The listing builds one solid part. Answer for the finished solid, in the listing's coordinates (mm). Round coordinates to 2 decimals unless told otherwise and drop trailing zeros. Put each result on its own line as item: value. Start each with the question number.
(1) Section A-A, the plane z = 999 is taken. Count the separate pieces of the cut face and the enclosed holes in it, then the cut area to 3 significant figures.
(2) Straight lines are drawn through the part: line 1 (Y direction, x = 27.4, z = 1000); line 2 (X direction, y = -50, z = 1000.5); line 3 (Y direction, x = -28, z = 999.65). For each, find the intervals that lie inside material, in ascending order.
(3) A flat-ended cylindrical pin translates along its axis: P1, Ø2, axis at x = 27.4, y = 15.47, coming from the -Z side. Find the tip coordinate at first contact, or state that the pin passes through.
```python
from build123d import *

# Parameters (mm, degrees)
CROQUIS1_W              = 110.308657865
CROQUIS1_H              = 110.308657866
CROQUIS1_R              = 3
SALIENTE_EXTRUIR1_DEPTH = 3
CROQUIS3_R              = 1.35
CORTAR_EXTRUIR1_DEPTH   = 4
SKETCH2_R               = 1.55575
CUT_EXTRUDE1_DEPTH      = 4
SKETCH1_R               = 1.1
CUT_EXTRUDE2_DEPTH      = 4


with BuildPart() as part:
    # Croquis1 → Saliente-Extruir1 (new body)
    with BuildSketch(Plane(origin=(25.025391454, -7.129133069, 1001.5), x_dir=(1, 0, 0), z_dir=(0, 0, 1))):
        with Locations((-25.025391455, 7.129133069)):
            Rectangle(CROQUIS1_W, CROQUIS1_H)
        with Locations((-74.389051931, 56.197819511)):
            Circle(CROQUIS1_R, mode=Mode.SUBTRACT)
        with Locations((24.605897435, -42.797129855)):
            Circle(CROQUIS1_R, mode=Mode.SUBTRACT)
        with Locations((-74.389051931, -42.797129855)):
            Circle(CROQUIS1_R, mode=Mode.SUBTRACT)
        with Locations((24.605897435, 56.197819511)):
            Circle(CROQUIS1_R, mode=Mode.SUBTRACT)
    extrude(amount=-SALIENTE_EXTRUIR1_DEPTH)

    # Croquis3 → Cortar-Extruir1 (cut, through all)
    with BuildSketch(Plane(origin=(25.025391454, -7.129133069, 998.5), x_dir=(-1, 0, 0), z_dir=(0, 0, -1))):
        with Locations((37.910718234, 21.399287334)):
            Circle(CROQUIS3_R)
        with Locations((37.910718234, -27.600712666)):
            Circle(CROQUIS3_R)
        with Locations((-20.089281766, -27.600712666)):
            Circle(CROQUIS3_R)
        with Locations((-20.089281766, 21.399287334)):
            Circle(CROQUIS3_R)
    extrude(amount=-CORTAR_EXTRUIR1_DEPTH, mode=Mode.SUBTRACT)

    # Sketch2 → Cut-Extrude1 (cut, through all)
    with BuildSketch(Plane(origin=(25.025391454, -7.129133069, 998.5), x_dir=(-1, 0, 0), z_dir=(0, 0, -1))):
        with Locations((30.006327248, 14.907883069)):
            Circle(SKETCH2_R)
        with Locations((30.006327248, -0.649616931)):
            Circle(SKETCH2_R)
    extrude(amount=-CUT_EXTRUDE1_DEPTH, mode=Mode.SUBTRACT)

    # Sketch1 → Cut-Extrude2 (cut, through all)
    with BuildSketch(Plane(origin=(25.025391454, -7.129133069, 998.5), x_dir=(-1, 0, 0), z_dir=(0, 0, -1))):
        with Locations((-2.374608546, 22.599287334)):
            Circle(SKETCH1_R)
        with Locations((10.125391454, 22.599287334)):
            Circle(SKETCH1_R)
        with Locations((10.125391454, 1.599287334)):
            Circle(SKETCH1_R)
        with Locations((-2.374608546, 1.599287334)):
            Circle(SKETCH1_R)
        with BuildLine():
            Line((50.625391454, 24.599287334), (53.625391454, 24.599287334))
            ThreePointArc((53.625391454, 24.599287334), (54.332498236, 24.306394115), (54.625391454, 23.599287334))
            Line((54.625391454, 23.599287334), (54.625391454, 0.599287334))
            ThreePointArc((54.625391454, 0.599287334), (54.332498236, -0.107819447), (53.625391454, -0.400712666))
            Line((53.625391454, -0.400712666), (50.625391454, -0.400712666))
            ThreePointArc((50.625391454, -0.400712666), (49.918284673, -0.107819447), (49.625391454, 0.599287334))
            Line((49.625391454, 0.599287334), (49.625391454, 23.599287334))
            ThreePointArc((49.625391454, 23.599287334), (49.918284673, 24.306394115), (50.625391454, 24.599287334))
        make_face()
    extrude(amount=-CUT_EXTRUDE2_DEPTH, mode=Mode.SUBTRACT)


solid = part.part
```
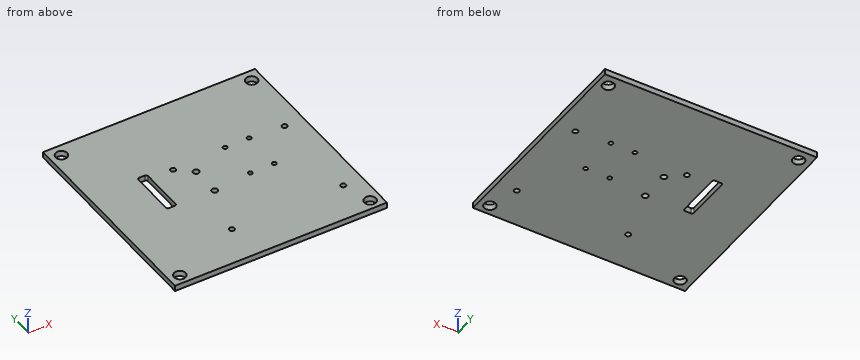
Recorded:
1. separate pieces: 1
1. enclosed holes: 15
1. area: 11,900 mm²
2. line 1: y = -55.15 to -6.63, -4.43 to 14.37, 16.57 to 55.15
2. line 2: x = -55.15 to -52.36, -46.36 to 46.63, 52.63 to 55.15
2. line 3: y = -55.15 to -7.53, 17.47 to 55.15
3. P1: passes through
